from build123d import *

# Parameters (mm, degrees)
SKETCH1_R           = 19
BOSS_EXTRUDE1_DEPTH = 6
SKETCH3_R           = 14.86
BOSS_EXTRUDE2_DEPTH = 2
SKETCH2_R           = 2.75
CUT_EXTRUDE1_DEPTH  = 10


with BuildPart() as part:
    # Sketch1 → Boss-Extrude1 (new body)
    with BuildSketch(Plane(origin=(0, 0, 0), x_dir=(1, 0, 0), z_dir=(0, 1, 0))):
        with BuildLine():
            ThreePointArc((-4, 39), (0, 43), (4, 39))
            Line((4, 39), (0, 39))
            Line((0, 39), (-4, 39))
        make_face()
        with BuildLine():
            ThreePointArc((-4, 18.574175621), (-2.011300972, 18.893243988), (0, 19))
            Line((0, 19), (0, 39))
            Line((0, 39), (-4, 39))
            Line((-4, 39), (-4, 18.574175621))
        make_face()
        with BuildLine():
            Line((0, 39), (0, 19))
            ThreePointArc((0, 19), (2.011300972, 18.893243988), (4, 18.574175621))
            Line((4, 18.574175621), (4, 39))
            Line((4, 39), (0, 39))
        make_face()
        Circle(SKETCH1_R)
    extrude(amount=BOSS_EXTRUDE1_DEPTH)

    # Sketch3 → Boss-Extrude2 (add)
    with BuildSketch(Plane.XZ):
        with Locations(Location((0, 0, 0), (0, 0, 90))):
            Circle(SKETCH3_R)
    extrude(amount=BOSS_EXTRUDE2_DEPTH)

    # Sketch2 → Cut-Extrude1 (cut)
    with BuildSketch(Plane(origin=(0, 6, 0), x_dir=(1, 0, 0), z_dir=(0, 1, 0))):
        with Locations(Location((8, 0, 0), (0, 0, 270))):
            Circle(SKETCH2_R)
        with Locations(Location((-8, 0, 0), (0, 0, 270))):
            Circle(SKETCH2_R)
    extrude(amount=-CUT_EXTRUDE1_DEPTH, mode=Mode.SUBTRACT)


solid = part.part
Check sheet for the modelled part. Datum: model origin and axes. Units: mm. A direction names the side the tool comes from. Give positions to 0.01 mm unless a question says otherwise; leave off trailing zeros. Loops run counter-clockwise (first coordinate to the right, second up) from the corner with the lowest first, then second, coordinate; pieces in that order, holes last. Notation, with made-up numbers: M 80,-19 L 99,-19 A9 ccw 99,-5 Z; hole C 24,2.25 d3. An arc over 180 degrees is marked long. Return JSON: item names as keys, results as strings. Group by question number.
1. Cross-section at B-B on y = 4.5. Record the boundary of the cut face in (x, z), plus the area to 3 significant figures.
2. Tool access check on faces 1 (the cylindrical face through (-12.53, -0.99, 7.99)), 2 (the flat face through (4, 3, -29)), 3 (the flat face through (-4, 3, -29)). Record the directions out of +Z, -Z, +X, -X, +Y, -Y that give a thin tool (end or side, any length) a straight path to the whole face; none if there is none.
3. Thickness scan on L1, parallel to X at y = 3.75, z = 0; L2, parallel to X at y = 4, z = -24; L3, parallel to Y at x = -2, z = -31. Record the ranges inside material, lowest first.
4. Cross-section at A-A on z = 0. Record the boundary of the cut face in (x, y), plus the area to 3 significant figures.
5. Go/stop test with flat-tipped pins: pin 1 (6 mm diameter, centred on x = -15, z = -3, fed in from -Y); pin 2 (19 mm diameter, centred on x = -2, z = -26.5, fed in from -Y); pin 3 (1.8 mm diameter, centred on y = 3, z = -32, fed in from -X); pin 4 (1.8 mm diameter, centred on y = 2, z = -28, fed in from +X). Record where each tip stops, or that it passes through.
6. Cross-section at C-C on x = 8. Record the boundary of the cut face in (y, z), plus the area to 3 significant figures.
7. Cross-section at D-D on z = -10.5. Record the boundary of the cut face in (x, y), plus the area to 3 significant figures.
8. Mould release check, pull along Z, two halves, no side actions. Record for faces 4 (the cylindrical face through (10.727, 2.056, -0.358)), 5 (the flat face through (0, -2, 0)), 6 (the cylindrical face through (-10.685, 2.056, -0.596)), 7 (the cylindrical face through (-0.779, 2.958, 18.984)): released by +Z, released by -Z, zero draft, split by the parting line, or undercut.
Return value:
{
 "1": {"outline": "M -4,-39 A4 ccw 4,-39 L 4,-18.57 A19 ccw long -4,-18.57 Z; hole C -8,0 d5.5; hole C 8,0 d5.5", "area": "1,270 mm^2"},
 "2": {"face 1": "-Y", "face 2": "-Z, +X, +Y, -Y", "face 3": "-Z, -X, +Y, -Y"},
 "3": {"L1": "-19 to -10.75, -5.25 to 5.25, 10.75 to 19", "L2": "-4 to 4", "L3": "0 to 6"},
 "4": {"outline": "M -19,0 L -14.86,0 L -14.86,-2 L -10.75,-2 L -10.75,6 L -19,6 Z; M -5.25,-2 L 5.25,-2 L 5.25,6 L -5.25,6 Z; M 10.75,-2 L 14.86,-2 L 14.86,0 L 19,0 L 19,6 L 10.75,6 Z", "area": "199 mm^2"},
 "5": {"pin 1": "y = -2", "pin 2": "y = 0", "pin 3": "x = -4", "pin 4": "x = 4"},
 "6": {"outline": "M -2,-12.52 L 0,-12.52 L 0,-17.23 L 6,-17.23 L 6,-2.75 L -2,-2.75 Z; M -2,2.75 L 6,2.75 L 6,17.23 L 0,17.23 L 0,12.52 L -2,12.52 Z", "area": "213 mm^2"},
 "7": {"outline": "M -15.84,0 L -10.52,0 L -10.52,-2 L 10.52,-2 L 10.52,0 L 15.84,0 L 15.84,6 L -15.84,6 Z", "area": "232 mm^2"},
 "8": {"face 4": "undercut", "face 5": "zero draft", "face 6": "undercut", "face 7": "split by the parting line"}
}
